Source: three-view drawing plus pictorial views. Frame: mm from the lowest corner of the part. A direction names the side the tool comes from. Round coordinates to 2 decimals unless told otherwise and drop trailing zeros. Loops run counter-clockwise (first coordinate to the right, second up) from the corner with the lowest first, then second, coordinate; pieces in that order, holes last. Notation, with made-up numbers: M 6.25,45.25 L 59.25,45.25 A27 cw 59.25,62.25 Z; hole C 38,79.25 d9. An arc over 180 degrees is marked long. Write each question's results on one line, items separated by ' | '.
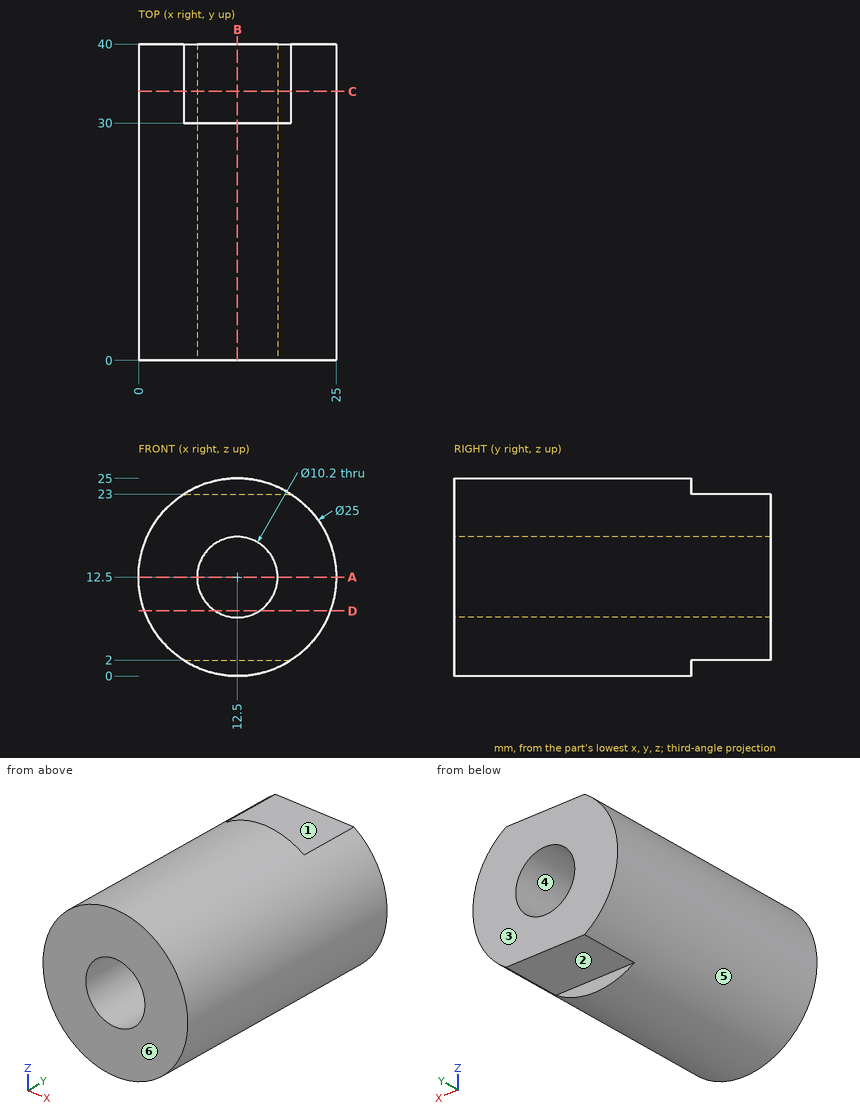
1. Section B-B (x = 12.5). Output: boundary loops of the cut face in (y, z), then the cut area to 3 significant figures.
Answer key:
outline: M 0,0 L 30,0 L 30,2 L 40,2 L 40,7.4 L 0,7.4 Z; M 0,17.6 L 40,17.6 L 40,23 L 30,23 L 30,25 L 0,25 Z | area: 552 mm²
2. Section C-C (y = 34). Output: boundary loops of the cut face in (x, z), then the cut area to 3 significant figures.
Answer key:
outline: M 5.72,2 L 19.28,2 A12.5 ccw 19.28,23 L 5.72,23 A12.5 ccw Z; hole C 12.5,12.5 d10.2 | area: 372 mm²
3. Section D-D (z = 8.25). Output: boundary loops of the cut face in (x, y), then the cut area to 3 significant figures.
Answer key:
outline: M 0.74,0 L 9.68,0 L 9.68,40 L 0.74,40 Z; M 15.32,0 L 24.26,0 L 24.26,40 L 15.32,40 Z | area: 715 mm²
4. Pin query (flat end, axial travel): P1, Ø1, axis at x = 10, y = 19.5, coming from the +Z side; P2, Ø1, axis at x = 13.5, z = 1, coming from the +Y side; P3, Ø1.5, axis at x = 14.5, y = 28, coming from the -Z side. Return the tip coordinate at first contact, or that it passes through.
Answer key:
P1: stops at z = 24.84 | P2: stops at y = 30 | P3: stops at z = 0.06
5. Section A-A (z = 12.5). Output: boundary loops of the cut face in (x, y), then the cut area to 3 significant figures.
Answer key:
outline: M 0,0 L 7.4,0 L 7.4,40 L 0,40 Z; M 17.6,0 L 25,0 L 25,40 L 17.6,40 Z | area: 592 mm²
6. Access query for the marked faces 1, 2 and 3. Directions: +Z, -Z, +X, -X, +Y, -Y. A direction counts if a zero-diameter tool reaches every point of the face in a straight line with its end or side. Return the directions, or none.
Answer key:
face 1: +Z, +X, -X, +Y | face 2: -Z, +X, -X, +Y | face 3: +Z, -Z, +X, -X, +Y
7. Draft query along X for the marked faces 4, 5 and 6. Return one class per face: pulls with the +X half, pulls with the -X half, needs draft (parallel to the pull), parting line crosses it, or undercut.
Answer key:
face 4: undercut | face 5: parting line crosses it | face 6: needs draft
8. Ray query, probe 1 along Z at (x, y) = (12.5, 21); probe 2 along Z at (x, y) = (9.25, 27); probe 3 along X at (y, z) = (30.5, 16.75). Return the intervals inside material, ascending.
Answer key:
probe 1: z = 0 to 7.4, 17.6 to 25 | probe 2: z = 0.43 to 8.57, 16.43 to 24.57 | probe 3: x = 0.74 to 9.68, 15.32 to 24.26
